Can you work these out from the model? Positions are in its coordinate system, mm. A direction names the side the tool comes from. Give positions to 0.01 mm unless a question says otherwise; leave off trailing zeros. Write each loop counter-clockwise with the first axis right and the second up, starting at its lowest first coordinate (ties: lowest second). Pieces come first, ordered by that corner, then holes.
from build123d import *

# Parameters (mm, degrees)
SALIENTE_EXTRUIR1_DEPTH = 2.5
CROQUIS2_R              = 1.45
CORTAR_EXTRUIR1_DEPTH   = 2.5
REDONDEO1_R             = 2


with BuildPart() as part:
    # Croquis1 → Saliente-Extruir1 (new body)
    with BuildSketch(Plane.XY):
        Polygon((0, 0), (0, 45), (53, 45), (53, 0), (36.5, 0), (36.5, 20), (21.5, 20), (21.5, 0), align=None)
    extrude(amount=SALIENTE_EXTRUIR1_DEPTH)

    # Croquis2 → Cortar-Extruir1 (cut)
    with BuildSketch(Plane.XY.offset(2.5)):
        with Locations((37.05, 29.354509915)):
            Circle(CROQUIS2_R)
        with Locations((21.65, 29.354509915)):
            Circle(CROQUIS2_R)
    extrude(amount=-CORTAR_EXTRUIR1_DEPTH, mode=Mode.SUBTRACT)

    # Redondeo1
    redondeo1_edges = [part.edges().sort_by_distance(p)[0] for p in [
        (0, 0, 1.25),
        (53, 45, 1.25),
        (53, 0, 1.25),
        (36.5, 0, 1.25),
        (36.5, 20, 1.25),
        (21.5, 20, 1.25),
        (21.5, 0, 1.25),
    ]]
    fillet(redondeo1_edges, radius=REDONDEO1_R)


solid = part.part
(1) Imagine slicing it at A-A, the plane y = 10. Write out the boundary of the cut face in (x, z).
Returned:
outline: (0, 0) - (21.5, 0) - (21.5, 2.5) - (0, 2.5) - close; (36.5, 0) - (53, 0) - (53, 2.5) - (36.5, 2.5) - close
(2) Imagine slicing it at C-C, the plane x = 31. Write out the boundary of the cut face in (y, z), plus the area to 3 significant figures.
Returned:
outline: (20, 0) - (45, 0) - (45, 2.5) - (20, 2.5) - close
area: 62.5 mm2
(3) If we mould it in two halves opening along X, with no side actions, what happens to faces 3 (the face through (27, 23, 2.5)), 4 (the face through (52.43, 0.6, 1.27)), 5 (the face through (29, 20, 1))? For each: +X half, -X half, draft (parallel to the pull), parting line (faces both ways), or undercut.
Returned:
face 3: draft
face 4: +X half
face 5: undercut
(4) Imagine slicing it at B-B, the plane z = 0.75. Write out the boundary of the cut face in (x, y), plus the area to 3 significant figures.
Returned:
outline: (0, 2) arc R2 ccw to (2, 0) - (19.5, 0) arc R2 ccw to (21.5, 2) - (21.5, 18) arc R2 cw to (23.5, 20) - (34.5, 20) arc R2 cw to (36.5, 18) - (36.5, 2) arc R2 ccw to (38.5, 0) - (51, 0) arc R2 ccw to (53, 2) - (53, 43) arc R2 ccw to (51, 45) - (0, 45) - close; hole circle Ø2.9 at (21.65, 29.35); hole circle Ø2.9 at (37.05, 29.35)
area: 2,070 mm2
(5) If I drill on L1, parallel to X at y = 29.5, z = 0.8; L2, parallel to X at y = 16, z = 0.7; L3, parallel to X at y = 19.5, z = 2.1, over which ranges is the centre line in solid material (lowest first)?
Returned:
L1: x = 0 to 20.21, 23.09 to 35.61, 38.49 to 53
L2: x = 0 to 21.5, 36.5 to 53
L3: x = 0 to 22.18, 35.82 to 53
(6) For faces 1 (the face through (37.1, 0.57, 1.27)), 2 (the face through (21.46, 30.79, 1.27)), which set-ups out of +Z, -Z, +X, -X, +Y, -Y let a thin tool reach every point of the face, with its end or its side?
Returned:
face 1: +Z, -Z, -Y
face 2: +Z, -Z
(7) Will this pin go through, and if not, where does the flat tip stop? P1, Ø0.8, axis at x = 31.5, z = 1.5, coming from the -Y side.
Returned:
P1: stops at y = 20
